Build history of the part. All positions in model axes, mm. A direction names the side the tool comes from. Coordinates: 2 decimals unless noted, no trailing zeros. Write each loop counter-clockwise with the first axis right and the second up, starting at its lowest first coordinate (ties: lowest second). Pieces come first, ordered by that corner, then holes. Notation, with made-up numbers: (-33, 17.5) -> (-24, 17.5) arc R8 ccw to (-24, 30.5) -> close; hole circle Ø9 at (59, 86.25). An arc over 180 degrees is marked (long way). Write each question's results on one line, items separated by ' | '. Start each with the question number.
Q1. Drill centre lines: line 1 (Y direction, x = -15.5, z = 6.9); line 2 (Y direction, x = -15.5, z = 2.1). Where is each one in solid material? Low to high.
Q2. Saw through at B-B on y = 52.5. Give the cut face in (x, z), and give its area (3 significant figures).
Q3. Two-plate mould, pull along Y, no slides. Class faces 1 (the face through (15.272, 17.235, 5.972)), 2 (the face through (-2, 21, 5)), 3 (the face through (-21, 1, 5)): released by +Y, released by -Y, zero draft, split by the parting line, or undercut.
Q4. Tool access for faces 4 (the face through (-12.267, 16.841, 1.972)), 5 (the face through (21, -2, 5)), 6 (the face through (19.52, 19.37, 2.2)): list every direction of +Z, -Z, +X, -X, +Y, -Y with a clear straight run to the whole face (end or side of a thin tool).
Q5. Saw through at C-C on x = 25.5. Give the cut face in (y, z).
Q6. Drop flat-ended pins along their axis: pin 1 Ø1.5 at (x, y) = (-41, -40) entering from +Z; pin 2 Ø5.5 at (x, y) = (15.5, -15.5) entering from -Z. Give the stop position or say it passes through.
Q7. Saw through at A-A on z = 6. Give the cut face in (x, y), and give its area (3 significant figures).
Q8. Saw through at D-D on y = 15.5. Give the cut face in (x, z), and give its area (3 significant figures).
from build123d import *

# Parameters (mm, degrees)
F0_W      = 42
F0_H      = 42
F0_R      = 1.75
F0_R_2    = 11.5
F1_DEPTH  = 5
F0_W_2    = 120
F0_H_2    = 120
F2_DEPTH  = 2
F4_DEPTH  = 2
F5_DEPTH  = 3
F6_R      = 3.5
F6_R_2    = 1.75
F7_DEPTH  = 4
F8_R      = 3.5
F8_R_2    = 1.75
F9_DEPTH  = 4
F10_R     = 3.5
F10_R_2   = 1.75
F11_DEPTH = 4
F12_DEPTH = 3
F14_DEPTH = 2
F15_DEPTH = 8


with BuildPart() as f1:
    # F0 (on Top) → F1 (new body)
    with BuildSketch(Plane.XY):
        Rectangle(F0_W, F0_H)
        with Locations((-15.5, -15.5)):
            Circle(F0_R, mode=Mode.SUBTRACT)
        with Locations((15.5, -15.5)):
            Circle(F0_R, mode=Mode.SUBTRACT)
        with Locations((-15.5, 15.5)):
            Circle(F0_R, mode=Mode.SUBTRACT)
        Circle(F0_R_2, mode=Mode.SUBTRACT)
        with Locations((15.5, 15.5)):
            Circle(F0_R, mode=Mode.SUBTRACT)
    extrude(amount=F1_DEPTH)

    # F0 (on Top) → F2 (join)
    with BuildSketch(Plane.XY):
        Rectangle(F0_W_2, F0_H_2)
        Rectangle(F0_W, F0_H, mode=Mode.SUBTRACT)
    extrude(amount=F2_DEPTH)

    # F3 (on face) → F4 (cut)
    with BuildSketch(Plane(origin=(0, 0, 0), x_dir=(1, 0, 0), z_dir=(0, 0, -1))):
        with BuildLine():
            Line((0, 27.5), (0, 55))
            ThreePointArc((0, 55), (-38.8908729653, 38.8908729653), (-55, 0))
            Line((-55, 0), (-27.5, 0))
            ThreePointArc((-27.5, 0), (-19.4454364826, 19.4454364826), (0, 27.5))
        make_face()
    extrude(amount=-F4_DEPTH, mode=Mode.SUBTRACT)

    # F5 (cut): a face of the model
    f5_faces = [f1.faces().sort_by_distance(p)[0] for p in [
        (-19.9487472991, -19.9487472991, 2),
    ]]
    extrude(f5_faces, amount=-F5_DEPTH, mode=Mode.SUBTRACT)

    # F6 (on face) → F7 (cut)
    with BuildSketch(Plane(origin=(0, 0, 0), x_dir=(1, 0, 0), z_dir=(0, 0, -1))):
        with Locations((-15.5, 15.5)):
            Circle(F6_R)
        with Locations((-15.5, 15.5)):
            Circle(F6_R_2, mode=Mode.SUBTRACT)
    extrude(amount=-F7_DEPTH, mode=Mode.SUBTRACT)

    # F8 (on face) → F9 (cut)
    with BuildSketch(Plane(origin=(0, 0, 0), x_dir=(1, 0, 0), z_dir=(0, 0, -1))):
        with Locations((15.5, 15.5)):
            Circle(F8_R)
        with Locations((15.5, 15.5)):
            Circle(F8_R_2, mode=Mode.SUBTRACT)
    extrude(amount=-F9_DEPTH, mode=Mode.SUBTRACT)

    # F10 (on face) → F11 (cut)
    with BuildSketch(Plane(origin=(0, 0, 0), x_dir=(1, 0, 0), z_dir=(0, 0, -1))):
        with Locations((-15.5, -15.5)):
            Circle(F10_R)
        with Locations((-15.5, -15.5)):
            Circle(F10_R_2, mode=Mode.SUBTRACT)
        with Locations((15.5, -15.5)):
            Circle(F10_R)
        with Locations((15.5, -15.5)):
            Circle(F10_R_2, mode=Mode.SUBTRACT)
    extrude(amount=-F11_DEPTH, mode=Mode.SUBTRACT)

    # F12 (add): a face of the model
    f12_faces = [f1.faces().sort_by_distance(p)[0] for p in [
        (1.6223595477, -20.4060303038, 5),
    ]]
    extrude(f12_faces, amount=F12_DEPTH)

    # F13 (on face) → F14 (cut)
    with BuildSketch(Plane(origin=(0, 0, 0), x_dir=(1, 0, 0), z_dir=(0, 0, -1))):
        with BuildLine():
            ThreePointArc((0, -55), (38.8908729653, -38.8908729653), (55, 0))
            Line((55, 0), (27.5, 0))
            ThreePointArc((27.5, 0), (19.4454364826, -19.4454364826), (0, -27.5))
            Line((0, -27.5), (0, -55))
        make_face()
    extrude(amount=-F14_DEPTH, mode=Mode.SUBTRACT)

    # F15 (cut): a face of the model
    f15_faces = [f1.faces().sort_by_distance(p)[0] for p in [
        (19.9487472991, 19.9487472991, 2),
    ]]
    extrude(f15_faces, amount=-F15_DEPTH, mode=Mode.SUBTRACT)


solid = f1.part
Returned:
1) line 1: y = -21 to -17.25, -13.75 to 13.75, 17.25 to 21 | line 2: y = -21 to -19, -12 to 12, 19 to 21
2) outline: (-60, 0) -> (0, 0) -> (0, 2) -> (-60, 2) -> close; (16.39, 0) -> (60, 0) -> (60, 2) -> (16.39, 2) -> close | area: 207 mm2
3) face 1: undercut | face 2: released by +Y | face 3: zero draft
4) face 4: -Z | face 5: +Z, +X, +Y, -Y | face 6: +Z, -Z
5) outline: (-60, 0) -> (10.3, 0) -> (10.3, 2) -> (-60, 2) -> close; (48.73, 0) -> (60, 0) -> (60, 2) -> (48.73, 2) -> close
6) pin 1: stops at z = 2 | pin 2: stops at z = 4
7) outline: (-21, -17.76) arc R27.5 ccw to (-17.76, -21) -> (21, -21) -> (21, 17.76) arc R27.5 ccw to (17.76, 21) -> (-21, 21) -> close; hole circle Ø3.5 at (-15.5, -15.5); hole circle Ø3.5 at (-15.5, 15.5); hole circle Ø23 at (0, 0); hole circle Ø3.5 at (15.5, -15.5); hole circle Ø3.5 at (15.5, 15.5) | area: 1,300 mm2
8) outline: (-60, 0) -> (-19, 0) -> (-19, 4) -> (-17.25, 4) -> (-17.25, 8) -> (-21, 8) -> (-21, 2) -> (-60, 2) -> close; (-13.75, 4) -> (-12, 4) -> (-12, 0) -> (12, 0) -> (12, 4) -> (13.75, 4) -> (13.75, 8) -> (-13.75, 8) -> close; (17.25, 4) -> (19, 4) -> (19, 0) -> (22.72, 0) -> (22.72, 2) -> (21, 2) -> (21, 8) -> (17.25, 8) -> close; (52.77, 0) -> (60, 0) -> (60, 2) -> (52.77, 2) -> close | area: 348 mm2
